Input: part model. Units: mm. Frame: model coordinates. Face numbers are marked on the shaded views. A direction names the side the tool comes from. Coordinates: 2 decimals unless noted, no trailing zeros. Loops run counter-clockwise (first coordinate to the right, second up) from the corner with the lowest first, then second, coordinate; pieces in that order, holes last.
```python
from build123d import *

# Parameters (mm, degrees)
SKETCH006_R     = 1.6
PAD003_DEPTH    = 22.5
SKETCH023_W     = 224
SKETCH023_H     = 224
POCKET006_DEPTH = 10
SKETCH025_R     = 23
POCKET007_DEPTH = 22.5
FILLET_R        = 2
FILLET010_R     = 3.6


with BuildPart() as part:
    # Sketch006 (on Face23 of Pad) → Pad003 (new body, symmetric)
    with BuildSketch(Plane(origin=(0, 0, -2), x_dir=(1, 0, 0), z_dir=(0, 0, -1))):
        with BuildLine():
            Line((-111.4, -3.8), (-15.556349, -3.8))
            ThreePointArc((-3.8, -15.556349), (-7.243355, -7.243355), (-15.556349, -3.8))
            Line((-3.8, -111.4), (-3.8, -15.556349))
            Line((3.8, -111.4), (-3.8, -111.4))
            Line((3.8, -111.4), (3.8, -15.556349))
            ThreePointArc((15.556349, -3.8), (7.243355, -7.243355), (3.8, -15.556349))
            Line((111.4, -3.8), (15.556349, -3.8))
            Line((111.4, -3.8), (111.4, 3.8))
            Line((111.4, 3.8), (15.556349, 3.8))
            ThreePointArc((3.8, 15.556349), (7.243355, 7.243355), (15.556349, 3.8))
            Line((3.8, 111.4), (3.8, 15.556349))
            Line((-3.8, 111.4), (3.8, 111.4))
            Line((-3.8, 111.4), (-3.8, 15.556349))
            ThreePointArc((-15.556349, 3.8), (-7.243355, 7.243355), (-3.8, 15.556349))
            Line((-111.4, 3.8), (-15.556349, 3.8))
            Line((-111.4, 3.8), (-111.4, -3.8))
        make_face()
        with Locations((-16.5, 0)):
            Circle(SKETCH006_R, mode=Mode.SUBTRACT)
        with Locations((0, -16.5)):
            Circle(SKETCH006_R, mode=Mode.SUBTRACT)
        with Locations((16.5, 0)):
            Circle(SKETCH006_R, mode=Mode.SUBTRACT)
        with Locations((0, 16.5)):
            Circle(SKETCH006_R, mode=Mode.SUBTRACT)
    extrude(amount=PAD003_DEPTH, both=True)

    # Sketch023 → Pocket006 (cut)
    with BuildSketch(Plane(origin=(0, 0, -24.5), x_dir=(1, 0, 0), z_dir=(0, 0, -1))):
        Rectangle(SKETCH023_W, SKETCH023_H)
    extrude(amount=-POCKET006_DEPTH, mode=Mode.SUBTRACT)

    # Sketch025 → Pocket007 (cut)
    with BuildSketch(Plane.XY.offset(20.5)):
        Circle(SKETCH025_R)
    extrude(amount=-POCKET007_DEPTH, mode=Mode.SUBTRACT)

    # Fillet
    fillet_edges = [part.edges().sort_by_distance(p)[0] for p in [
        (0, -23, -2),
        (0, 23, -2),
        (22.920843, 1.906562, -2),
        (-23, 0, -2),
    ]]
    fillet(fillet_edges, radius=FILLET_R)

    # Fillet010
    fillet010_edges = [part.edges().sort_by_distance(p)[0] for p in [
        (0, 23, 20.5),
        (3.8, 67.041958, 20.5),
        (0, 111.4, 20.5),
        (-3.8, 67.041958, 20.5),
        (67.041958, -3.8, 20.5),
        (111.4, 0, 20.5),
        (67.041958, 3.8, 20.5),
        (22.920843, 1.906562, 20.5),
        (22.920843, -1.906562, 20.5),
        (-3.8, -67.041958, 20.5),
        (0, -111.4, 20.5),
        (3.8, -67.041958, 20.5),
        (0, -23, 20.5),
        (-67.041958, -3.8, 20.5),
        (-23, 0, 20.5),
        (-67.041958, 3.8, 20.5),
        (-111.4, 0, 20.5),
    ]]
    fillet(fillet010_edges, radius=FILLET010_R)


solid = part.part
```
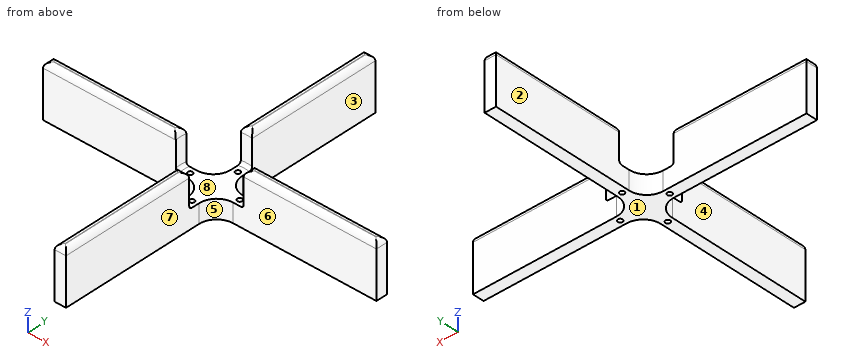
Item 1: Section query B-B (z = -11.5). Output: boundary loops of the cut face in (x, y), then the cut area to 3 significant figures.
Result:
outline: (-111.4, -3.8) - (-15.56, -3.8) arc R11.76 cw to (-3.8, -15.56) - (-3.8, -111.4) - (3.8, -111.4) - (3.8, -15.56) arc R11.76 cw to (15.56, -3.8) - (111.4, -3.8) - (111.4, 3.8) - (15.56, 3.8) arc R11.76 cw to (3.8, 15.56) - (3.8, 111.4) - (-3.8, 111.4) - (-3.8, 15.56) arc R11.76 cw to (-15.56, 3.8) - (-111.4, 3.8) - close; hole circle Ø3.2 at (-16.5, 0); hole circle Ø3.2 at (0, -16.5); hole circle Ø3.2 at (0, 16.5); hole circle Ø3.2 at (16.5, 0)
area: 3,420 mm2
Item 2: Section query C-C (x = -47.5). Output: boundary loops of the cut face in (y, z), then the cut area to 3 significant figures.
Result:
outline: (-3.8, -14.5) - (3.8, -14.5) - (3.8, 16.9) arc R3.6 ccw to (0.2, 20.5) - (-0.2, 20.5) arc R3.6 ccw to (-3.8, 16.9) - close
area: 260 mm2
Item 3: Contact query for flat-ended pins moving along their axis: P1, Ø6, axis at y = 42.5, z = -2, coming from the -X side; P2, Ø3.5, axis at x = -16.5, y = 0, coming from the +Z side; P3, Ø2, axis at x = -57, z = 7, coming from the +Y side; P4, Ø1.9, axis at x = 0, y = 16.5, coming from the -Z side. Output: stop coordinate, or through.
Result:
P1: stops at x = -3.8
P2: stops at z = -2
P3: stops at y = 3.8
P4: passes through
Item 4: Section query A-A (z = 14). Output: boundary loops of the cut face in (x, y), then the cut area to 3 significant figures.
Result:
outline: (-111.4, -3.8) - (-22.68, -3.8) arc R23 cw to (-22.68, 3.8) - (-111.4, 3.8) - close; (-3.8, -111.4) - (3.8, -111.4) - (3.8, -22.68) arc R23 cw to (-3.8, -22.68) - close; (-3.8, 22.68) arc R23 cw to (3.8, 22.68) - (3.8, 111.4) - (-3.8, 111.4) - close; (22.68, -3.8) - (111.4, -3.8) - (111.4, 3.8) - (22.68, 3.8) arc R23 cw to start
area: 2,690 mm2
Item 5: Line query: L1, parallel to Y at x = 0, z = -8; L2, parallel to Y at x = -16.5, z = -9.25; L3, parallel to X at y = 51, z = -10. Output: solid intervals per line, ascending.
Result:
L1: y = -111.4 to -18.1, -14.9 to 14.9, 18.1 to 111.4
L2: y = -3.8 to -1.6, 1.6 to 3.8
L3: x = -3.8 to 3.8
Item 6: Reachability of the marked faces 1, 2, 3, 4 and 5 from +Z, -Z, +X, -X, +Y, -Y: full face, straight path, thin tool, end or side. Return the list, or none.
Result:
face 1: -Z, +X, -X, +Y, -Y
face 2: +Z, -Z, -X, +Y
face 3: +Z, -Z, +X, +Y
face 4: +Z, -Z, -X, -Y
face 5: +Z, -Z, +X, -Y
Item 7: Mould query, pull axis X, two halves, no side actions, for the marked faces 6, 7 and 8. Classes: +X half, -X half, draft (parallel to the pull), parting line (faces both ways), or undercut.
Result:
face 6: draft
face 7: +X half
face 8: undercut
